from build123d import *

# Parameters (mm, degrees)
BOSS_EXTRUDE1_DEPTH      = 1
SKETCH11_W               = 12
SKETCH11_H               = 5
CUT_EXTRUDE7_DEPTH       = 10
SKETCH13_R               = 3
CUT_EXTRUDE9_DEPTH       = 10
CUT_EXTRUDE10_DEPTH      = 10
SKETCH21_R               = 6.5
CUT_EXTRUDE11_DEPTH      = 10
CUT_EXTRUDE17_DEPTH      = 10
CUT_EXTRUDE17_DEPTH_BACK = 10
SKETCH23_W               = 2
SKETCH23_H               = 4
BOSS_EXTRUDE2_DEPTH      = 3
SKETCH24_W               = 2
SKETCH24_H               = 3.949234692
BOSS_EXTRUDE3_DEPTH      = 3
FILLET1_R                = 2
SKETCH25_R               = 0.5
CUT_EXTRUDE18_DEPTH      = 10


with BuildPart() as part:
    # Sketch4 → Boss-Extrude1 (new body)
    with BuildSketch(Plane.XY):
        with BuildLine():
            Line((55, 14.052488348), (0, 14.052488348))
            Line((0, 14.052488348), (-55, 14.052488348))
            ThreePointArc((-55, 14.052488348), (-58.535533906, 12.588022254), (-60, 9.052488348))
            Line((-60, 9.052488348), (-60, -8.947511652))
            ThreePointArc((-60, -8.947511652), (-58.535533906, -12.483045558), (-55, -13.947511652))
            Line((-55, -13.947511652), (0, -13.947511652))
            Line((0, -13.947511652), (55, -13.947511652))
            ThreePointArc((55, -13.947511652), (58.535533906, -12.483045558), (60, -8.947511652))
            Line((60, -8.947511652), (60, 9.052488348))
            ThreePointArc((60, 9.052488348), (58.535533906, 12.588022254), (55, 14.052488348))
        make_face()
    extrude(amount=BOSS_EXTRUDE1_DEPTH)

    # Sketch11 → Cut-Extrude7 (cut)
    with BuildSketch(Plane.XY.offset(1)):
        with Locations((4, 3.552488348)):
            Rectangle(SKETCH11_W, SKETCH11_H)
    extrude(amount=-CUT_EXTRUDE7_DEPTH, mode=Mode.SUBTRACT)

    # Sketch13 → Cut-Extrude9 (cut)
    with BuildSketch(Plane.XY.offset(1)):
        with Locations((46.180246868, 4.878767266)):
            Circle(SKETCH13_R)
    extrude(amount=-CUT_EXTRUDE9_DEPTH, mode=Mode.SUBTRACT)

    # Sketch12 → Cut-Extrude10 (cut)
    with BuildSketch(Plane.XY.offset(1)):
        with BuildLine():
            Line((38.300111452, -2.809077948), (32.100111452, -2.809077948))
            ThreePointArc((32.100111452, -2.809077948), (31.746558061, -2.955524558), (31.600111452, -3.309077948))
            Line((31.600111452, -3.309077948), (31.600111452, -5.309077948))
            Line((31.600111452, -5.309077948), (38.800111452, -5.309077948))
            Line((38.800111452, -5.309077948), (38.800111452, -3.309077948))
            ThreePointArc((38.800111452, -3.309077948), (38.653664842, -2.955524558), (38.300111452, -2.809077948))
        make_face()
    extrude(amount=-CUT_EXTRUDE10_DEPTH, mode=Mode.SUBTRACT)

    # Sketch21 → Cut-Extrude11 (cut)
    with BuildSketch(Plane.XY.offset(1)):
        with Locations((22.972397633, 2.485770253)):
            Circle(SKETCH21_R)
    extrude(amount=-CUT_EXTRUDE11_DEPTH, mode=Mode.SUBTRACT)

    # Sketch22 → Cut-Extrude17 (cut, two sides: drawn at the far end of the back side and taken through both)
    with BuildSketch(Plane.XY.offset(-CUT_EXTRUDE17_DEPTH_BACK)):
        with BuildLine():
            Line((-39.794789509, -7.812631563), (-39.794789509, -10.545937078))
            Line((-39.794789509, -10.545937078), (-37.794789509, -10.545937078))
            Line((-37.794789509, -10.545937078), (-37.794789509, -1.545937078))
            Line((-37.794789509, -1.545937078), (-39.794789509, -1.545937078))
            Line((-39.794789509, -1.545937078), (-39.794789509, -4.279242592))
            ThreePointArc((-39.794789509, -4.279242592), (-45.219411252, -6.045937078), (-39.794789509, -7.812631563))
        make_face()
        with BuildLine():
            Line((-25.510698687, -1.545937078), (-23.510698687, -1.545937078))
            Line((-23.510698687, -1.545937078), (-23.510698687, -4.279242592))
            ThreePointArc((-23.510698687, -4.279242592), (-18.086076945, -6.045937078), (-23.510698687, -7.812631563))
            Line((-23.510698687, -7.812631563), (-23.510698687, -10.545937078))
            Line((-23.510698687, -10.545937078), (-25.510698687, -10.545937078))
            Line((-25.510698687, -10.545937078), (-25.510698687, -1.545937078))
        make_face()
        with BuildLine():
            Line((-31.652744098, 3.313523563), (-34.652744098, 3.313523563))
            Line((-34.652744098, 3.313523563), (-34.652744098, 7.397933855))
            ThreePointArc((-34.652744098, 7.397933855), (-31.652744098, 10.397933855), (-28.652744098, 7.397933855))
            Line((-28.652744098, 7.397933855), (-28.652744098, 3.313523563))
            Line((-28.652744098, 3.313523563), (-31.652744098, 3.313523563))
        make_face()
    extrude(amount=CUT_EXTRUDE17_DEPTH + CUT_EXTRUDE17_DEPTH_BACK, mode=Mode.SUBTRACT)

    # Sketch23 → Boss-Extrude2 (add)
    with BuildSketch(Plane(origin=(0, 0, 0), x_dir=(-1, 0, 0), z_dir=(0, 0, -1))):
        with Locations((-55.128215007, 1.148016517)):
            Rectangle(SKETCH23_W, SKETCH23_H)
    extrude(amount=BOSS_EXTRUDE2_DEPTH)

    # Sketch24 → Boss-Extrude3 (add)
    with BuildSketch(Plane(origin=(0, 0, 0), x_dir=(-1, 0, 0), z_dir=(0, 0, -1))):
        with Locations((55.13, 1.173399171)):
            Rectangle(SKETCH24_W, SKETCH24_H)
    extrude(amount=BOSS_EXTRUDE3_DEPTH)

    # Fillet1
    # the kernel refuses this fillet: 2 mm, written as the material it takes off along each edge
    with BuildSketch(Plane(origin=(22.972397633, 2.485770253, 1), x_dir=(1, 0, 0), z_dir=(0, -1, 0))) as fillet1_piece_1:
        with BuildLine():
            CenterArc((8.232050808, -2), FILLET1_R, 90, 60)
            Line((6.5, -1), (6.465358984, -0.98))
            ThreePointArc((6.465358984, -0.98), (6.46, -0.5), (6.46, 0))
            Line((6.46, 0), (6.5, 0.04))
            Line((6.5, 0.04), (8.232050808, 0.04))
            Line((8.232050808, 0.04), (8.232050808, 0))
        make_face()
    revolve(axis=Axis((22.972397633, 2.485770253, 1), (0, 0, 1)), mode=Mode.SUBTRACT)

    # Sketch25 → Cut-Extrude18 (cut)
    with BuildSketch(Plane.XY.offset(1)):
        with Locations((46.180246868, -2.877511652)):
            Circle(SKETCH25_R)
    extrude(amount=-CUT_EXTRUDE18_DEPTH, mode=Mode.SUBTRACT)


solid = part.part
Check sheet for the modelled part. Datum: model origin and axes. Units: mm. A direction names the side the tool comes from. Round coordinates to 2 decimals unless told otherwise and drop trailing zeros. Write each loop counter-clockwise with the first axis right and the second up, starting at its lowest first coordinate (ties: lowest second). Pieces come first, ordered by that corner, then holes. Notation, with made-up numbers: (19.5, 70.25) -> (23.5, 70.25) arc R9 cw to (23.5, 84.25) -> close; hole circle Ø6 at (8.5, -19). An arc over 180 degrees is marked (long way). Answer as CSV lines item,"result". Start each with the question number.
1) Material ranges on line 1 (Y direction, x = 5.5, z = 0.8); line 2 (X direction, y = 6.25, z = 0.2); line 3 (X direction, y = 0.75, z = -0.15), recorded low to high. Write a range as from..to.
2) Section check D-D on y = -12. Enter the section's corners in (x, z), and give its area (3 significant figures).
3) Section check C-C on x = -48. Enter the section's corners in (y, z), and give its area (3 significant figures).
4) Section check B-B on x = 1. Enter the section's corners in (y, z).
5) Release check for a two-part mould opening along X. For faces 4 (the cylindrical face through (-18.088, -5.94, 0.493)), 5 (the flat face through (55, -0.852, -1)), 6 (the flat face through (-56.13, 1, -1)) record: pulls with the +X half, pulls with the -X half, needs draft (parallel to the pull), parting line crosses it, or undercut.
6) Go/stop test with flat-tipped pins: P1, Ø2, axis at x = 13.5, y = 5, coming from the -Z side; P2, Ø0.6, axis at x = -55.5, z = -1.5, coming from the -Y side. Record where each tip stops, or that it passes through.
7) Section check A-A on z = -1.95. Enter the section's corners in (x, y).
8) Tool access check on faces 1 (the flat face through (-55, 3.148, -1)), 2 (the flat face through (-54.13, 1, -1)), 3 (the flat face through (56.128, 1, -1)). Record the directions out of +Z, -Z, +X, -X, +Y, -Y that give a thin tool (end or side, any length) a straight path to the whole face; none if there is none.
Found:
1,line 1,"y = -13.95..1.05, 6.05..14.05"
1,line 2,"x = -60..-34.65, -28.65..17.51, 28.43..43.51, 48.85..60"
1,line 3,"x = -56.13..-54.13, 54.13..56.13"
2,outline,"(-58.96, 0) -> (58.96, 0) -> (58.96, 1) -> (-58.96, 1) -> close"
2,area,"118 mm^2"
3,outline,"(-13.95, 0) -> (14.05, 0) -> (14.05, 1) -> (-13.95, 1) -> close"
3,area,"28.0 mm^2"
4,outline,"(-13.95, 0) -> (1.05, 0) -> (1.05, 1) -> (-13.95, 1) -> close; (6.05, 0) -> (14.05, 0) -> (14.05, 1) -> (6.05, 1) -> close"
5,face 4,"undercut"
5,face 5,"needs draft"
5,face 6,"pulls with the -X half"
6,P1,"stops at z = 0"
6,P2,"stops at y = -0.8"
7,outline,"(-56.13, -0.8) -> (-54.13, -0.8) -> (-54.13, 3.15) -> (-56.13, 3.15) -> close; (54.13, -0.85) -> (56.13, -0.85) -> (56.13, 3.15) -> (54.13, 3.15) -> close"
8,face 1,"-Z, +X, -X, +Y"
8,face 2,"-Z, +Y, -Y"
8,face 3,"-Z, +X, +Y, -Y"
